from build123d import *

# Parameters (mm, degrees)
BOSS_EXTRUDE1_DEPTH = 22
SKETCH2_R           = 3.05
SKETCH2_W           = 5
SKETCH2_H           = 5
CUT_EXTRUDE1_DEPTH  = 24.248655875
FILLET1_R           = 0.25
FILLET2_R           = 0.5


with BuildPart() as part:
    # Sketch1 → Boss-Extrude1 (new body)
    with BuildSketch(Plane(origin=(0, 0, 0), x_dir=(1, 0, 0), z_dir=(0, 1, 0))):
        Polygon((3.7, 0.3), (3.7, -1.2), (-3.7, -1.2), (-3.7, 0.3), (-5.7, 0.3), (-5.7, 3.7), (5.7, 3.7), (5.7, 0.3), align=None)
    extrude(amount=-BOSS_EXTRUDE1_DEPTH)

    # Sketch2 → Cut-Extrude1 (cut, through all)
    with BuildSketch(Plane.XY.offset(1.2)):
        with Locations((0, -6)):
            Circle(SKETCH2_R)
        with Locations((0, -14.5)):
            Rectangle(SKETCH2_W, SKETCH2_H)
    extrude(amount=-CUT_EXTRUDE1_DEPTH, mode=Mode.SUBTRACT)

    # Fillet1
    fillet1_edges = [part.edges().sort_by_distance(p)[0] for p in [
        (3.7, -11, -0.3),
        (-3.7, -11, -0.3),
        (-5.7, -11, -0.3),
        (-5.7, -11, -3.7),
        (5.7, -11, -3.7),
        (5.7, -11, -0.3),
    ]]
    fillet(fillet1_edges, radius=FILLET1_R)

    # Fillet2
    fillet2_edges = [part.edges().sort_by_distance(p)[0] for p in [
        (2.5, -12, -1.25),
        (2.5, -17, -1.25),
        (-2.5, -17, -1.25),
        (-2.5, -12, -1.25),
    ]]
    fillet(fillet2_edges, radius=FILLET2_R)


solid = part.part
Part model, mm, in its own coordinate system. A direction names the side the tool comes from. Round coordinates to 2 decimals unless told otherwise and drop trailing zeros. Write each loop counter-clockwise with the first axis right and the second up, starting at its lowest first coordinate (ties: lowest second). Pieces come first, ordered by that corner, then holes. Notation, with made-up numbers: (11.25, -2) - (38.25, -2) arc R28 ccw to (38.25, 26) - close; hole circle Ø9 at (62, 62). An arc over 180 degrees is marked (long way). Use CSV: the item, a comma, the result in double quotes.
Item 1: Pull direction Y, two halves, no side cores. Call faces 5 (the flat face through (-2.5, -15, -1)), 6 (the flat face through (0, -22, -1)), 7 (the flat face through (0, -11, 1.2)): pulls with the +Y half, pulls with the -Y half, needs draft (parallel to the pull), parting line crosses it, or undercut.
Results list:
face 5,"undercut"
face 6,"pulls with the -Y half"
face 7,"needs draft"
Item 2: Tool access for faces 1 (the flat face through (-5, -11, -0.3)), 2 (the flat face through (0, -12, -1)), 3 (the flat face through (5, -11, -0.3)), 4 (the flat face through (-5.7, -11, -2)): list every direction of +Z, -Z, +X, -X, +Y, -Y with a clear straight run to the whole face (end or side of a thin tool).
Results list:
face 1,"+Z, -X, +Y, -Y"
face 2,"+Z, -Z"
face 3,"+Z, +X, +Y, -Y"
face 4,"+Z, -Z, -X, +Y, -Y"
Item 3: Slice it at C-C, the plane z = -1.6. Write the cut outline in (x, y).
Results list:
outline,"(-5.7, -22) - (5.7, -22) - (5.7, 0) - (-5.7, 0) - close; hole circle Ø6.1 at (0, -6); hole (-2.5, -16.5) arc R0.5 ccw to (-2, -17) - (2, -17) arc R0.5 ccw to (2.5, -16.5) - (2.5, -12.5) arc R0.5 ccw to (2, -12) - (-2, -12) arc R0.5 ccw to (-2.5, -12.5) - close"
Item 4: Wall check: L1, parallel to Y at x = 0, z = 0; L2, parallel to Y at x = 1, z = -0.3; L3, parallel to X at y = -16.25, z = -0.8. Give the ranges that are in metal, low to high.
Results list:
L1,"y = -22 to -17, -12 to -9.05, -2.95 to 0"
L2,"y = -22 to -17, -12 to -8.88, -3.12 to 0"
L3,"x = -5.7 to -2.5, 2.5 to 5.7"
Item 5: Slice it at D-D, the plane x = -2.75. Write the cut outline in (y, z).
Results list:
outline,"(-22, -3.7) - (-7.32, -3.7) - (-7.32, 1.2) - (-22, 1.2) - close; (-4.68, -3.7) - (0, -3.7) - (0, 1.2) - (-4.68, 1.2) - close"
Item 6: Slice it at A-A, the plane y = -6. Write the cut outline in (x, z).
Results list:
outline,"(-5.7, -3.45) arc R0.25 ccw to (-5.45, -3.7) - (-3.05, -3.7) - (-3.05, 1.2) - (-3.7, 1.2) - (-3.7, -0.05) arc R0.25 cw to (-3.95, -0.3) - (-5.45, -0.3) arc R0.25 ccw to (-5.7, -0.55) - close; (3.05, -3.7) - (5.45, -3.7) arc R0.25 ccw to (5.7, -3.45) - (5.7, -0.55) arc R0.25 ccw to (5.45, -0.3) - (3.95, -0.3) arc R0.25 cw to (3.7, -0.05) - (3.7, 1.2) - (3.05, 1.2) - close"
Item 7: Flat gauge pins, fed straight in: P1, Ø0.6, axis at y = -8, z = 0.5, coming from the +X side; P2, Ø1, axis at x = -1.5, y = -14, coming from the +Z side; P3, Ø1.2, axis at x = 0.5, z = -2, coming from the +Y side; P4, Ø1.4, axis at y = -6, z = 1, coming from the -X side. Where does each tip first touch, or does it go through?
Results list:
P1,"stops at x = 3.7"
P2,"passes through"
P3,"stops at y = 0"
P4,"stops at x = -3.7"
Item 8: Slice it at B-B, the plane x = 0. Write the cut outline in (y, z).
Results list:
outline,"(-22, -3.7) - (-17, -3.7) - (-17, 1.2) - (-22, 1.2) - close; (-12, -3.7) - (-9.05, -3.7) - (-9.05, 1.2) - (-12, 1.2) - close; (-2.95, -3.7) - (0, -3.7) - (0, 1.2) - (-2.95, 1.2) - close"
